from build123d import *

# Parameters (mm, degrees)
F0_W     = 35.890091
F0_H     = 39.142508
F1_DEPTH = 50.8
F2_R     = 14.892015
F3_DEPTH = 50.8
F4_R     = 14.730043
F5_DEPTH = 12.7
F6_W     = 21.786809
F6_H     = 22.704257
F7_DEPTH = 12.7


with BuildPart() as f1:
    # F0 (on Front) → F1 (new body)
    with BuildSketch(Plane.XZ):
        with Locations((32.447086, 19.571254)):
            Rectangle(F0_W, F0_H)
    extrude(amount=F1_DEPTH)

    # F2 (on face) → F3 (cut)
    with BuildSketch(Plane.XZ.offset(50.8)):
        with Locations((32.93968, 18.618079)):
            Circle(F2_R)
    extrude(amount=-F3_DEPTH, mode=Mode.SUBTRACT)

    # F4 (on face) → F5 (join)
    with BuildSketch(Plane(origin=(14.502041, 0, 0), x_dir=(0, -1, 0), z_dir=(-1, 0, 0))):
        with Locations((24.537444, 20.065336)):
            Circle(F4_R)
    extrude(amount=F5_DEPTH)

    # F6 (on face) → F7 (join)
    with BuildSketch(Plane.XY.offset(39.142508)):
        with Locations((33.557378, -23.779297)):
            Rectangle(F6_W, F6_H)
    extrude(amount=F7_DEPTH)


solid = f1.part
Can you work these out from the model? Positions are in its coordinate system, mm. A direction names the side the tool comes from. Coordinates: 2 decimals unless noted, no trailing zeros. Order: outer loops, then holes, each group sorted by start corner. A loop starts at its lowest first (then second) coordinate and runs counter-clockwise, first axis right, second up. Notation, with made-up numbers: M 83.25,-26 L 135.25,-26 A24 ccw 135.25,8 Z; hole C -17.5,7.5 d2. An arc over 180 degrees is marked long. Write item = value, one per line.
(1) Suppose I cut it at D-D on x = 20. Please give me the cut outline in (y, z), plus the area to 3 significant figures.
Results are:
outline = M -50.8,0 L 0,0 L 0,11.25 L -50.8,11.25 Z; M -50.8,25.99 L 0,25.99 L 0,39.14 L -50.8,39.14 Z
area = 1,240 mm2
(2) For pin 1 Ø12 at (x, y) = (21.5, -40.5) entering from -Z; pin 2 Ø24 at (x, z) = (32.94, 18.62) entering from -Y; pin 3 Ø4 at (y, z) = (-20.5, 43.5) entering from -X; pin 4 Ø6.5 at (x, z) = (39, 45) entering from -Y, each with a flat end and sliding along its axis, tell me the tip position at first contact or that it passes through.
Results are:
pin_1 = 0
pin_2 = through
pin_3 = 22.66
pin_4 = -35.13
(3) If we mould it in two halves opening along Z, with no side actions, what happens to faces 1 (the face through (28, -50.8, 33)), 2 (the face through (40.946, -25.756, 31.175)), 3 (the face through (32, -25, 0))? For each: pulls with the +Z half, pulls with the -Z half, needs draft (parallel to the pull), parting line crosses it, or undercut.
Results are:
face_1 = needs draft
face_2 = undercut
face_3 = pulls with the -Z half
(4) Suppose I cut it at B-B on x = 32.5. Please give me the cut outline in (y, z).
Results are:
outline = M -50.8,0 L 0,0 L 0,3.73 L -50.8,3.73 Z; M -50.8,33.5 L 0,33.5 L 0,39.14 L -12.43,39.14 L -12.43,51.84 L -35.13,51.84 L -35.13,39.14 L -50.8,39.14 Z
(5) Suppose I cut it at C-C on y = -36.5. Please give me the cut outline in (x, z).
Results are:
outline = M 1.8,11.47 L 14.5,11.47 L 14.5,0 L 50.39,0 L 50.39,39.14 L 14.5,39.14 L 14.5,28.66 L 1.8,28.66 Z; hole C 32.94,18.62 d29.78
(6) Suppose I cut it at A-A on z = 28.5. Please give me the cut outline in (x, y), plus the area to 3 significant figures.
Results are:
outline = M 1.8,-36.61 L 14.5,-36.61 L 14.5,-50.8 L 21.8,-50.8 L 21.8,0 L 14.5,0 L 14.5,-12.46 L 1.8,-12.46 Z; M 44.08,-50.8 L 50.39,-50.8 L 50.39,0 L 44.08,0 Z
area = 998 mm2
(7) I need wall thicknesses on line 1 along Z through (x, y) = (33.5, -15); line 2 along Y through (x, z) = (23.5, 49); line 3 along X through (y, z) = (-27, 11). Which ranges of each line are inside material? Lowest first, please. Write a range as [from, to].
Results are:
line_1 = [0, 3.74], [33.5, 51.84]
line_2 = [-35.13, -12.43]
line_3 = [1.8, 20.14], [45.74, 50.39]
(8) For faces 4 (the face through (33, -35.131, 45)), 5 (the face through (14.502, -31, 6)), 6 (the face through (22.664, -24, 45)), 7 (the face through (33, -12.427, 45)), which set-ups out of +Z, -Z, +X, -X, +Y, -Y let a thin tool reach every point of the face, with its end or its side?
Results are:
face_4 = +Z, +X, -X, -Y
face_5 = -X
face_6 = +Z, -X, +Y, -Y
face_7 = +Z, +X, -X, +Y
